Part model, mm, in its own coordinate system. Face numbers are marked on the shaded views. A direction names the side the tool comes from. Give positions to 0.01 mm unless a question says otherwise; leave off trailing zeros. Write each loop counter-clockwise with the first axis right and the second up, starting at its lowest first coordinate (ties: lowest second). Pieces come first, ordered by that corner, then holes. Notation, with made-up numbers: (-6.5, 19.5) - (20.5, 19.5) arc R21 cw to (20.5, 35.5) - close; hole circle Ø6 at (-38.5, 53.5). An arc over 180 degrees is marked (long way). Answer in a Markdown table with one row per item. Add a question column.
1. Which spindle directions (+Z, -Z, +X, -X, +Y, -Y) get a long thin tool onto all of the face, cutting with end or side? Do the marked faces 4 and 5. Say none if no direction does.
2. Probe line 1 along Y through (x, z) = (0, 19); line 2 along Y through (x, z) = (-4, 17.25); line 3 along Z through (x, y) = (6, -3.5). List the from-to ranges inside material, lowest first.
3. Pull direction X, two halves, no side cores. Call the marked faces 1, 2 and 3: released by +X, released by -X, zero draft, split by the parting line, or undercut.
4. Band-saw the part on B-B on z = 2.25. Write the cut outline in (x, y), plus the area to 3 significant figures.
5. Drop flat-ended pins along their axis: pin 1 Ø8 at (x, y) = (4, -12.5) entering from +Z; pin 2 Ø4 at (x, y) = (18, 0) entering from -Z; pin 3 Ø6 at (x, z) = (15.5, 21) entering from +Y. Give the stop position or say it passes through.
6. Band-saw the part on A-A on x = 0. Write the cut outline in (y, z).
7. Band-saw the part on C-C on z = 7.75. Write the cut outline in (x, y).
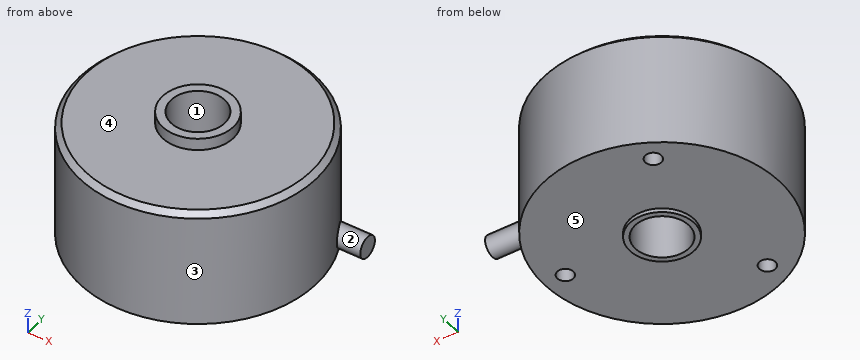
Autodesk Inventor part; units mm, degrees
ref_plane "YZ Plane" through (0, 0, 0) normal (1, 0, 0) x (0, 1, 0)
ref_plane "XZ Plane" through (0, 0, 0) normal (0, 1, 0) x (-1, 0, 0)
ref_plane "XY Plane" through (0, 0, 0) normal (0, 0, 1) x (1, 0, 0)
sketch "スケッチ1" plane through (0, 0, 0) normal (0, 0, 1) x (1, 0, 0)
  circle A0 centre (0, 0) radius 22
  dimension "d0" = 44
extrude "押し出し1" add sketch "スケッチ1" along normal blind 22
chamfer "面取り1" distance 1 angle 45 1 edges at (-22, 0, 22)
sketch "スケッチ2" plane through (0, 0, 22) normal (0, 0, 1) x (1, 0, 0)
  circle A0 centre (0, 0) radius 6.6
  dimension "d6" = 13.2
extrude "押し出し2" add sketch "スケッチ2" along normal blind 2.25
sketch "スケッチ6" plane through (0, 0, 0) normal (0, 0, 1) x (1, 0, 0)
  point P0 (0, 0)
sketch "スケッチ8" plane through (0, 0, 0) normal (0, 1, 0) x (-1, 0, 0)
  point P0 (0, 0)
sketch "スケッチ9" plane through (0, 0, 0) normal (1, 0, 0) x (0, 1, 0)
  line L0 (-22, 0) -> (22, 0)
  circle A0 centre (9.6776, 2.25) radius 2
  point P0 (0, 0)
  dimension "d30" = 2.25
  dimension "d31" = 4
extrude "押し出し3" add sketch "スケッチ9" along normal blind 25
sketch "スケッチ12" plane through (0, 0, 0) normal (0, 0, -1) x (-1, 0, 0)
  circle A0 centre (0, 0) radius 6
  dimension "d44" = 12
extrude "押し出し5" add sketch "スケッチ12" along normal blind 0.75
sketch "スケッチ13" plane through (0, 0, 24.25) normal (0, 0, 1) x (1, 0, 0)
  point P0 (0, 0)
  point P1 (0, 0)
hole "穴4" at (0, 0, 24.25) direction (0, 0, -1) diameter 10 end through all
sketch "スケッチ14" plane through (0, 0, 0) normal (0, 0, -1) x (-1, 0, 0)
  point P0 (0, 0)
  point P1 (-18, 0)
  point P2 (9, -15.5885)
  point P3 (9, 15.5885)
  dimension "d54" = 18
  dimension "d57" = 360
hole "穴5" at (18, 0, 0) at (-9, -15.5885, 0) at (-9, 15.5885, 0) direction (0, 0, 1) diameter 3 depth 5 tip angle 118
properties part number "meh-30-pエンコーダ"
Values:
| question | item | result |
|---|---|---|
| 1 | face 4 | +Z |
| 1 | face 5 | -Z |
| 2 | line 1 | y = -22 to -5, 5 to 22 |
| 2 | line 2 | y = -21.63 to -3, 3 to 21.63 |
| 2 | line 3 | z = 0 to 22 |
| 3 | face 1 | undercut |
| 3 | face 2 | zero draft |
| 3 | face 3 | split by the parting line |
| 4 | outline | (18.64, 11.68) arc R22 ccw (long way) to (20.62, 7.68) - (25, 7.68) - (25, 11.68) - close; hole circle Ø3 at (-9, -15.59); hole circle Ø3 at (-9, 15.59); hole circle Ø10 at (0, 0); hole circle Ø3 at (18, 0) |
| 4 | area | 1,440 mm² |
| 5 | pin 1 | stops at z = 22 |
| 5 | pin 2 | stops at z = 0 |
| 5 | pin 3 | stops at y = 18.1 |
| 6 | outline | (-22, 0) - (-6, 0) - (-6, -0.75) - (-5, -0.75) - (-5, 24.25) - (-6.6, 24.25) - (-6.6, 22) - (-21, 22) - (-22, 21) - close; (5, -0.75) - (6, -0.75) - (6, 0) - (22, 0) - (22, 21) - (21, 22) - (6.6, 22) - (6.6, 24.25) - (5, 24.25) - close |
| 7 | outline | circle Ø44 at (0, 0); hole circle Ø10 at (0, 0) |
